from build123d import *

# Parameters (mm, degrees)
F1_DEPTH = 30
F2_R     = 5
F3_R     = 2.5
F4_SIZE2 = 1
F4_SIZE  = 5
F5_R     = 4.7732777186
F6_DEPTH = 25.4


with BuildPart() as f1:
    # F0 (on Top) → F1 (new body)
    with BuildSketch(Plane.XY):
        with BuildLine():
            Line((8.6023872718, -25.1175931746), (-25.2596801519, -25.1175931746))
            Line((-25.2596801519, -25.1175931746), (-25.2596801519, -45.1175931746))
            Line((-25.2596801519, -45.1175931746), (24.7403198481, -45.1175931746))
            Line((24.7403198481, -45.1175931746), (24.7403198481, -25.1175931746))
            Line((24.7403198481, -25.1175931746), (21.1665723473, -25.1175931746))
            Line((21.1665723473, -25.1175931746), (18.9759883363, -29.909516218))
            ThreePointArc((18.9759883363, -29.909516218), (15.8660389828, -38.4984737312), (13.1416287482, -29.7795537856))
            Line((13.1416287482, -29.7795537856), (8.6023872718, -25.1175931746))
        make_face()
    extrude(amount=F1_DEPTH)

    # F2
    f2_edges = [f1.edges().sort_by_distance(p)[0] for p in [
        (-25.25968, -25.117593, 15),
        (-25.25968, -45.117593, 15),
        (24.74032, -45.117593, 15),
    ]]
    fillet(f2_edges, radius=F2_R)

    # F3
    f3_edges = [f1.edges().sort_by_distance(p)[0] for p in [
        (24.74032, -25.117593, 15),
        (8.602387, -25.117593, 15),
    ]]
    fillet(f3_edges, radius=F3_R)

    # F4
    f4_edges = [f1.edges().sort_by_distance(p)[0] for p in [
        (15.866039, -38.498474, 30),
    ]]
    f4_side = f1.faces().sort_by_distance((15.866039, -38.498474, 15))[0]
    chamfer(f4_edges, length=F4_SIZE, length2=F4_SIZE2, reference=f4_side)

    # F5 (on face) → F6 (cut)
    with BuildSketch(Plane.XY.offset(30)):
        with Locations((-12.9745947197, -35.1175931746)):
            Circle(F5_R)
    extrude(amount=-F6_DEPTH, mode=Mode.SUBTRACT)


solid = f1.part
Part model, mm, in its own coordinate system. A direction names the side the tool comes from. Round coordinates to 2 decimals unless told otherwise and drop trailing zeros. Loops run counter-clockwise (first coordinate to the right, second up) from the corner with the lowest first, then second, coordinate; pieces in that order, holes last. Notation, with made-up numbers: (36.25, -19) - (88.25, -19) arc R19 ccw to (88.25, 12) - close; hole circle Ø5 at (1.25, 81). An arc over 180 degrees is marked (long way). Answer as a JSON object with one key per item and string values.
Item 1: Band-saw the part on D-D on y = -43.5. List the corners of the cut face in (x, z), plus the area to 3 significant figures.
Output:
{"outline": "(-23.94, 0) - (23.42, 0) - (23.42, 30) - (-23.94, 30) - close", "area": "1,420 mm2"}
Item 2: Band-saw the part on C-C on z = 12. List the corners of the cut face in (x, y), plus the area to 3 significant figures.
Output:
{"outline": "(-25.26, -40.12) arc R5 ccw to (-20.26, -45.12) - (19.74, -45.12) arc R5 ccw to (24.74, -40.12) - (24.74, -27.62) arc R2.5 ccw to (22.24, -25.12) - (21.17, -25.12) - (18.98, -29.91) arc R4.82 cw (long way) to (13.14, -29.78) - (9.34, -25.87) arc R2.5 ccw to (7.55, -25.12) - (-20.26, -25.12) arc R5 ccw to (-25.26, -30.12) - close; hole circle Ø9.55 at (-12.97, -35.12)", "area": "798 mm2"}
Item 3: Tool access for faces 1 (the face through (-13, -35, 4.6)), 2 (the face through (20.087, -27.48, 14.79)), 3 (the face through (24.74, -34, 15)): list every direction of +Z, -Z, +X, -X, +Y, -Y with a clear straight run to the whole face (end or side of a thin tool).
Output:
{"face 1": "+Z", "face 2": "+Z, -Z, +Y", "face 3": "+Z, -Z, +X, +Y, -Y"}
Item 4: Pin check, flat tip, straight feed: pin 1 (5.5 mm diameter, centred on x = -12.97, y = -35.12, fed in from +Z). Stop position of the tip, or through.
Output:
{"pin 1": "z = 4.6"}
Item 5: Wall check: L1, parallel to X at y = -30.75, z = 27; L2, parallel to X at y = -38, z = 14; L3, parallel to Y at x = 12, z = 19. Give the ranges that are in metal, low to high.
Output:
{"L1": "-25.26 to -14.9, -11.05 to 11.65, 20.29 to 24.74", "L2": "-25.26 to -16.78, -9.17 to 13.84, 18.11 to 24.74", "L3": "-45.12 to -36.41, -30.95 to -28.61"}
Item 6: Band-saw the part on A-A on z = 3.5. List the corners of the cut face in (x, y), plus the area to 3 significant figures.
Output:
{"outline": "(-25.26, -40.12) arc R5 ccw to (-20.26, -45.12) - (19.74, -45.12) arc R5 ccw to (24.74, -40.12) - (24.74, -27.62) arc R2.5 ccw to (22.24, -25.12) - (21.17, -25.12) - (18.98, -29.91) arc R4.82 cw (long way) to (13.14, -29.78) - (9.34, -25.87) arc R2.5 ccw to (7.55, -25.12) - (-20.26, -25.12) arc R5 ccw to (-25.26, -30.12) - close", "area": "870 mm2"}
Item 7: Band-saw the part on B-B on x = -13.5. List the corners of the cut face in (y, z), plus the area to 3 significant figures.
Output:
{"outline": "(-45.12, 0) - (-25.12, 0) - (-25.12, 30) - (-30.37, 30) - (-30.37, 4.6) - (-39.86, 4.6) - (-39.86, 30) - (-45.12, 30) - close", "area": "359 mm2"}
Item 8: Pull direction X, two halves, no side cores. Call faces 4 (the face through (23.99, -25.83, 15.21)), 5 (the face through (-23.834, -43.614, 15.21)), 6 (the face through (-10.4, -31.1, 17.5)): pulls with the +X half, pulls with the -X half, needs draft (parallel to the pull), parting line crosses it, or undercut.
Output:
{"face 4": "pulls with the +X half", "face 5": "pulls with the -X half", "face 6": "undercut"}
